Model file for the job. Use its own axes, mm. Face numbers are marked on the shaded views. A direction names the side the tool comes from. Round coordinates to 2 decimals unless told otherwise and drop trailing zeros. Loops run counter-clockwise (first coordinate to the right, second up) from the corner with the lowest first, then second, coordinate; pieces in that order, holes last. Notation, with made-up numbers: M -15.75,18.5 L 40.25,18.5 A18 cw 40.25,43.5 Z; hole C 76,-22.5 d1. An arc over 180 degrees is marked long. Use a Markdown table: item, result. Add a question column.
Q1. Cut at C-C (z = 14.75). Give the cut face in (x, y) (3 decimals).
Q2. Cut at A-A (z = 5.75). Give the cut face in (x, y) (3 decimals), plus the area to 3 significant figures.
Q3. Pin check, flat tips, straight feed: pin 1 (2.5 mm diameter, centred on x = 1.5, y = 0, fed in from +Z) (3 decimals); pin 2 (13 mm diameter, centred on x = 0, y = 0, fed in from -Z); pin 3 (1.7 mm diameter, centred on x = -9.5, z = 16.5, fed in from +Y); pin 4 (2 mm diameter, centred on y = 1.5, z = 15, fed in from -X). Stop position of each tip, or through.
Q4. Tool access for the marked faces 3, 4 and 5: list every direction of +Z, -Z, +X, -X, +Y, -Y with a clear straight run to the whole face (end or side of a thin tool).
Q5. Probe line 1 (Y direction, x = 0, z = 5.5) (3 decimals); line 2 (X direction, y = -1.75, z = 7.5); line 3 (Y direction, x = 3, z = 11.75). List the from-to ranges inside material, lowest first. Write a range as from..to.
Q6. Mould opens along Y. For the marked faces 1 and 2 say: +Y half, -Y half, draft (parallel to the pull), parting line (faces both ways), or undercut.
Q7. Cut at D-D (x = -0.5). Give the cut face in (y, z) (1 decimal).
Q8. Cut at B-B (y = -1.75). Give the cut face in (x, z) (1 decimal).
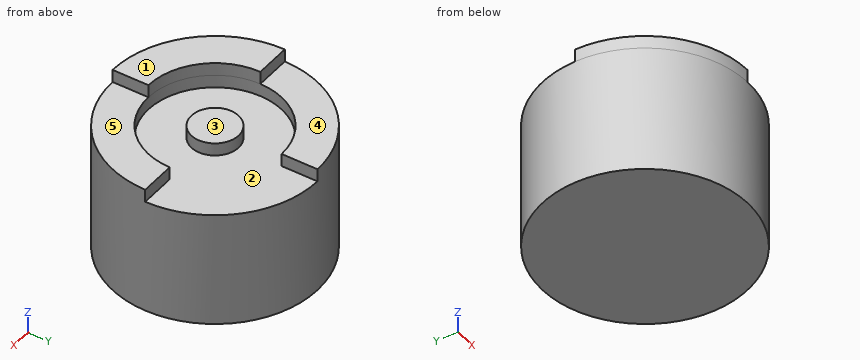
from build123d import *

# Parameters (mm, degrees)
F0_R      = 12.7
F0_R_2    = 8.255
F0_R_3    = 2.921
F1_DEPTH  = 15.875
F2_R      = 8.255
F2_R_2    = 2.921
F3_DEPTH  = 1.5875
F5_DEPTH  = 1.5875
F7_DEPTH  = 1.5875
F9_R      = 10.795
F9_R_2    = 8.255
F10_DEPTH = 9.525
F11_R     = 4.0925147824
F11_R_2   = 2.147201803
F12_DEPTH = 9.525


with BuildPart() as f1:
    # F0 (on Top) → F1 (new body)
    with BuildSketch(Plane.XY):
        Circle(F0_R)
        Circle(F0_R_2, mode=Mode.SUBTRACT)
        Circle(F0_R_2)
        Circle(F0_R_3, mode=Mode.SUBTRACT)
        Circle(F0_R_3)
    extrude(amount=F1_DEPTH)

    # F2 (on face) → F3 (cut)
    with BuildSketch(Plane.XY.offset(15.875)):
        Circle(F2_R)
        Circle(F2_R_2, mode=Mode.SUBTRACT)
    extrude(amount=-F3_DEPTH, mode=Mode.SUBTRACT)

    # F4 (on face) → F5 (cut, through all)
    with BuildSketch(Plane.XY.offset(15.875)):
        with BuildLine():
            ThreePointArc((0, 8.255), (5.8371664787, 5.8371664787), (8.255, 0))
            Line((8.255, 0), (12.7, 0))
            ThreePointArc((12.7, 0), (8.9802561211, 8.9802561211), (0, 12.7))
            Line((0, 12.7), (0, 8.255))
        make_face()
    extrude(amount=-F5_DEPTH, mode=Mode.SUBTRACT)

    # F6 (on face) → F7 (join)
    with BuildSketch(Plane.XY.offset(15.875)):
        with BuildLine():
            Line((0, -12.7), (0, -8.255))
            ThreePointArc((0, -8.255), (-5.8371664787, -5.8371664787), (-8.255, 0))
            Line((-8.255, 0), (-12.7, 0))
            ThreePointArc((-12.7, 0), (-8.9802561211, -8.9802561211), (0, -12.7))
        make_face()
    extrude(amount=F7_DEPTH)

    # F9 (on offset) → F10 (cut)
    with BuildSketch(Plane.XY.offset(2.54)):
        Circle(F9_R)
        Circle(F9_R_2, mode=Mode.SUBTRACT)
    extrude(amount=F10_DEPTH, mode=Mode.SUBTRACT)

    # F11 (on offset) → F12 (cut)
    with BuildSketch(Plane.XY.offset(2.54)):
        Circle(F11_R)
        Circle(F11_R_2, mode=Mode.SUBTRACT)
    extrude(amount=F12_DEPTH, mode=Mode.SUBTRACT)


solid = f1.part
Checked values:
| question | item | result |
|---|---|---|
| 1 | outline | C 0,0 d5.842; M 0,8.255 L 0,12.7 A12.7 ccw long 12.7,0 L 8.255,0 A8.255 cw long Z |
| 2 | outline | C 0,0 d25.4; C 0,0 d16.51; C 0,0 d4.294; hole C 0,0 d21.59; hole C 0,0 d8.185 |
| 2 | area | 317 mm^2 |
| 3 | pin 1 | stops at z = 15.875 |
| 3 | pin 2 | stops at z = 0 |
| 3 | pin 3 | stops at y = 9.04 |
| 3 | pin 4 | stops at x = -12.69 |
| 4 | face 3 | +Z, +X, +Y |
| 4 | face 4 | +Z, +X, -X, +Y |
| 4 | face 5 | +Z, +X, +Y, -Y |
| 5 | line 1 | y = -12.7..-10.795, -8.255..-4.093, -2.147..2.147, 4.093..8.255, 10.795..12.7 |
| 5 | line 2 | x = -12.58..-10.65, -8.07..-3.7, -1.24..1.24, 3.7..8.07, 10.65..12.58 |
| 5 | line 3 | y = -12.34..-10.37, -7.69..-2.78, 2.78..7.69, 10.37..12.34 |
| 6 | face 1 | draft |
| 6 | face 2 | undercut |
| 7 | outline | M -12.7,0 L 12.7,0 L 12.7,15.9 L 8.2,15.9 L 8.2,14.3 L 2.9,14.3 L 2.9,15.9 L -2.9,15.9 L -2.9,14.3 L -8.2,14.3 L -8.2,17.5 L -12.7,17.5 Z; hole M -10.8,2.5 L -8.2,2.5 L -8.2,12.1 L -10.8,12.1 Z; hole M -4.1,2.5 L -2.1,2.5 L -2.1,12.1 L -4.1,12.1 Z; hole M 2.1,2.5 L 4.1,2.5 L 4.1,12.1 L 2.1,12.1 Z; hole M 8.2,2.5 L 10.8,2.5 L 10.8,12.1 L 8.2,12.1 Z |
| 8 | outline | M -12.6,0 L 12.6,0 L 12.6,15.9 L 8.1,15.9 L 8.1,14.3 L 2.3,14.3 L 2.3,15.9 L -2.3,15.9 L -2.3,14.3 L -8.1,14.3 L -8.1,17.5 L -12.6,17.5 Z; hole M -10.7,2.5 L -8.1,2.5 L -8.1,12.1 L -10.7,12.1 Z; hole M -3.7,2.5 L -1.2,2.5 L -1.2,12.1 L -3.7,12.1 Z; hole M 1.2,2.5 L 3.7,2.5 L 3.7,12.1 L 1.2,12.1 Z; hole M 8.1,2.5 L 10.7,2.5 L 10.7,12.1 L 8.1,12.1 Z |
